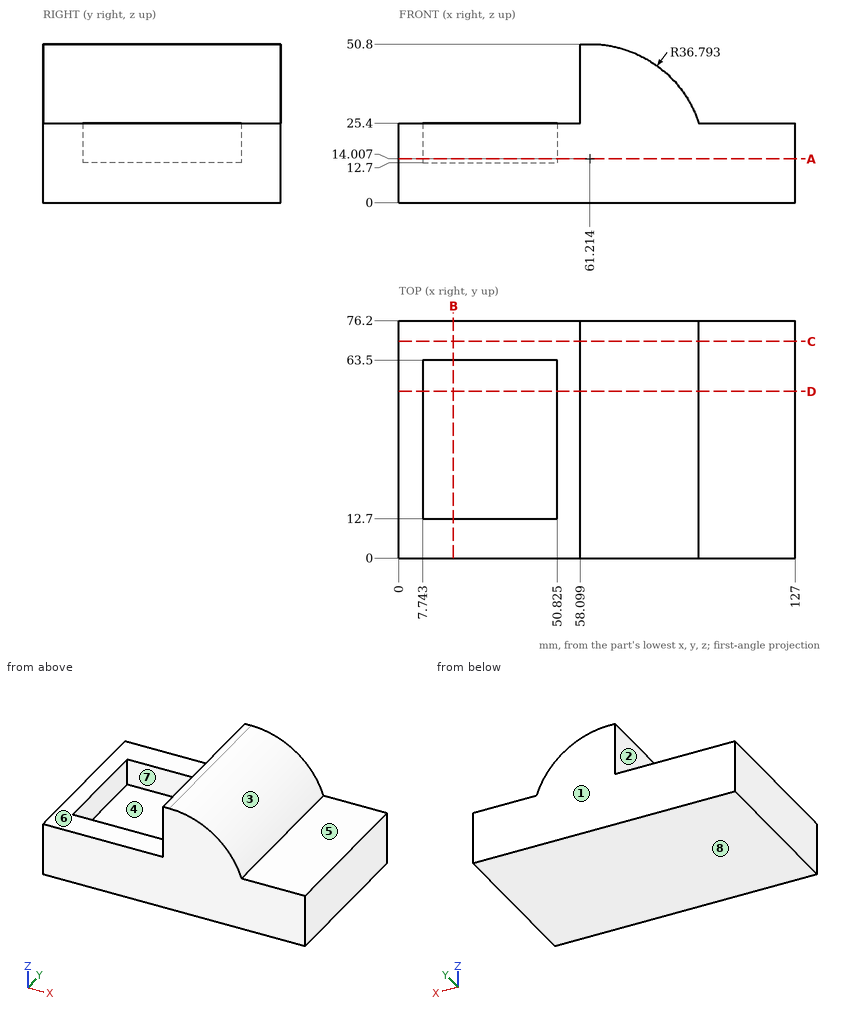
Part print with two shaded views. Sizes in mm from the minimum x, y, z corner. A direction names the side the tool comes from. Round coordinates to 2 decimals unless told otherwise and drop trailing zeros. Write each loop counter-clockwise with the first axis right and the second up, starting at its lowest first coordinate (ties: lowest second). Pieces come first, ordered by that corner, then holes. Notation, with made-up numbers: (63.25, 26) - (67.25, 26) arc R28 cw to (67.25, 58) - close; hole circle Ø1 at (20.25, -33.75). An arc over 180 degrees is marked (long way). Use CSV: the item, a comma, the result in double quotes.
Item 1: Slice it at B-B, the plane x = 17.5. Write the cut outline in (y, z).
Results list:
outline,"(0, 0) - (76.2, 0) - (76.2, 25.4) - (63.5, 25.4) - (63.5, 12.7) - (12.7, 12.7) - (12.7, 25.4) - (0, 25.4) - close"
Item 2: Slice it at C-C, the plane y = 69.5. Write the cut outline in (x, z) (1 decimal), then the cut area to 3 significant figures.
Results list:
outline,"(0, 0) - (127, 0) - (127, 25.4) - (96.2, 25.4) arc R36.8 ccw to (61.2, 50.8) - (58.1, 50.8) - (58.1, 25.4) - (0, 25.4) - close"
area,"3,960 mm²"
Item 3: Wall check: L1, parallel to Y at x = 22, z = 19.5; L2, parallel to Z at x = 15.5, y = 49; L3, parallel to Z at x = 53.5, y = 57. Give the ranges that are in metal, low to high.
Results list:
L1,"y = 0 to 12.7, 63.5 to 76.2"
L2,"z = 0 to 12.7"
L3,"z = 0 to 25.4"
Item 4: Tool access for the marked faces 5, 6, 7 and 8: list every direction of +Z, -Z, +X, -X, +Y, -Y with a clear straight run to the whole face (end or side of a thin tool).
Results list:
face 5,"+Z, +X, +Y, -Y"
face 6,"+Z, -X, +Y, -Y"
face 7,"+Z"
face 8,"-Z, +X, -X, +Y, -Y"
Item 5: Pull direction X, two halves, no side cores. Call the marked faces 1, 2, 3 and 4: pulls with the +X half, pulls with the -X half, needs draft (parallel to the pull), parting line crosses it, or undercut.
Results list:
face 1,"needs draft"
face 2,"pulls with the -X half"
face 3,"pulls with the +X half"
face 4,"undercut"
Item 6: Flat gauge pins, fed straight in: P1, Ø21.5, axis at x = 19.5, y = 43, coming from the +Z side; P2, Ø9, axis at x = 109, y = 30, coming from the +Z side; P3, Ø3, axis at y = 11, z = 42, coming from the -X side. Where does each tip first touch, or does it go through?
Results list:
P1,"stops at z = 12.7"
P2,"stops at z = 25.4"
P3,"stops at x = 58.1"
Item 7: Slice it at D-D, the plane y = 53.5. Write the cut outline in (x, z) (1 decimal), then the cut area to 3 significant figures.
Results list:
outline,"(0, 0) - (127, 0) - (127, 25.4) - (96.2, 25.4) arc R36.8 ccw to (61.2, 50.8) - (58.1, 50.8) - (58.1, 25.4) - (50.8, 25.4) - (50.8, 12.7) - (7.7, 12.7) - (7.7, 25.4) - (0, 25.4) - close"
area,"3,410 mm²"
Item 8: Slice it at A-A, the plane z = 14. Write the cut outline in (x, y) (1 decimal), then the cut area to 3 significant figures.
Results list:
outline,"(0, 0) - (127, 0) - (127, 76.2) - (0, 76.2) - close; hole (7.7, 12.7) - (50.8, 12.7) - (50.8, 63.5) - (7.7, 63.5) - close"
area,"7,490 mm²"
